Geometry check sheet. Reference: the model listing, model coordinates, mm. Round coordinates to 2 decimals unless told otherwise and drop trailing zeros. Order: outer loops, then holes, each group sorted by start corner. A loop starts at its lowest first (then second) coordinate and runs counter-clockwise, first axis right, second up. Notation, with made-up numbers: (16.25, 4.5) - (72.25, 4.5) arc R27 ccw to (72.25, 23.5) - close; hole circle Ø9 at (23, 76.5). An arc over 180 degrees is marked (long way). One line per question, with ' | ' between items. Start each with the question number.
Q1. Sectioned sample at B-B, the plane y = -26. Enter the section's corners in (x, z) (3 decimals), then the cut area to 3 significant figures.
Q2. Mould release check, pull along X, two halves, no side actions. Record for faces 1 (the face through (-52.175, 0, 13)), 2 (the face through (-22.29, 23.64, 12.97)), 3 (the face through (-1, -33.725, 13)), 4 (the face through (24.27, -22.12, 12.97)): +X half, -X half, draft (parallel to the pull), parting line (faces both ways), or undercut.
Q3. Gauge pin test, flat end, axial feed: P1, Ø3, axis at x = 24.6, y = 24.6, coming from the +Z side. Record the tip position at first contact, or that the pin passes through.
Q4. Sectioned sample at C-C, the plane z = 2. Give the number of separate pieces and of enclosed holes in the cut face, then the cut area to 3 significant figures.
Q5. Material ranges on line 1 along Y through (x, z) = (-24.6, 19.75) (3 decimals); line 2 along X through (y, z) = (24.6, 16.75) (3 decimals); line 3 along X through (y, z) = (-22, 12) (3 decimals), recorded low to high.
Q6. Sectioned sample at A-A, the plane x = 24.6. Enter the section's corners in (y, z) (3 decimals).
```python
from build123d import *

# Parameters (mm, degrees)
F0_W     = 104.35
F0_H     = 67.45
F1_DEPTH = 26.3
F2_R     = 2.5
F3_DEPTH = 26.301
F4_R     = 2
F5_DEPTH = 70.6


with BuildPart() as f1:
    # F0 (on Top) → F1 (new body)
    with BuildSketch(Plane.XY):
        Rectangle(F0_W, F0_H)
    extrude(amount=F1_DEPTH)

    # F2 (on Top) → F3 (cut, through all)
    with BuildSketch(Plane.XY):
        with Locations((-24.6, 24.6)):
            Circle(F2_R)
        with Locations((-24.6, -24.6)):
            Circle(F2_R)
        with Locations((24.6, -24.6)):
            Circle(F2_R)
        with Locations((24.6, 24.6)):
            Circle(F2_R)
    extrude(amount=F3_DEPTH, mode=Mode.SUBTRACT)

    # F4 (on Top) → F5 (cut)
    with BuildSketch(Plane.XY):
        with Locations((43.475, 20.225)):
            Circle(F4_R)
        with Locations((43.475, -20.225)):
            Circle(F4_R)
        with Locations((-37.925, 22.475)):
            Circle(F4_R)
        with Locations((-37.925, -22.475)):
            Circle(F4_R)
    extrude(amount=F5_DEPTH, mode=Mode.SUBTRACT)


solid = f1.part
```
Determined:
1) outline: (-52.175, 0) - (-26.671, 0) - (-26.671, 26.3) - (-52.175, 26.3) - close; (-22.529, 0) - (22.529, 0) - (22.529, 26.3) - (-22.529, 26.3) - close; (26.671, 0) - (52.175, 0) - (52.175, 26.3) - (26.671, 26.3) - close | area: 2,530 mm2
2) face 1: -X half | face 2: undercut | face 3: draft | face 4: undercut
3) P1: passes through
4) separate pieces: 1 | enclosed holes: 8 | area: 6,910 mm2
5) line 1: y = -33.725 to -27.1, -22.1 to 22.1, 27.1 to 33.725 | line 2: x = -52.175 to -27.1, -22.1 to 22.1, 27.1 to 52.175 | line 3: x = -52.175 to -39.868, -35.982 to 42.553, 44.397 to 52.175
6) outline: (-33.725, 0) - (-27.1, 0) - (-27.1, 26.3) - (-33.725, 26.3) - close; (-22.1, 0) - (22.1, 0) - (22.1, 26.3) - (-22.1, 26.3) - close; (27.1, 0) - (33.725, 0) - (33.725, 26.3) - (27.1, 26.3) - close
